from build123d import *

# Parameters (mm, degrees)
F0_R     = 9
F0_R_2   = 4.25
F1_DEPTH = 10
F2_SIZE2 = 0.3639702343
F2_SIZE  = 1
F3_SIZE2 = 0.3639702343
F3_SIZE  = 1
F4_SIZE2 = 0.3639702343
F4_SIZE  = 1
F5_SIZE2 = 0.3639702343
F5_SIZE  = 1


with BuildPart() as f1:
    # F0 (on Top) → F1 (new body)
    with BuildSketch(Plane.XY):
        Circle(F0_R)
        Circle(F0_R_2, mode=Mode.SUBTRACT)
    extrude(amount=F1_DEPTH)

    # F2
    f2_edges = [f1.edges().sort_by_distance(p)[0] for p in [
        (-4.25, 0, 10),
    ]]
    f2_side = f1.faces().sort_by_distance((-4.25, 0, 5))[0]
    chamfer(f2_edges, length=F2_SIZE, length2=F2_SIZE2, reference=f2_side)

    # F3
    f3_edges = [f1.edges().sort_by_distance(p)[0] for p in [
        (-9, 0, 10),
    ]]
    f3_side = f1.faces().sort_by_distance((-9, 0, 5))[0]
    chamfer(f3_edges, length=F3_SIZE, length2=F3_SIZE2, reference=f3_side)

    # F4
    f4_edges = [f1.edges().sort_by_distance(p)[0] for p in [
        (-9, 0, 0),
    ]]
    f4_side = f1.faces().sort_by_distance((-9, 0, 4.5))[0]
    chamfer(f4_edges, length=F4_SIZE, length2=F4_SIZE2, reference=f4_side)

    # F5
    f5_edges = [f1.edges().sort_by_distance(p)[0] for p in [
        (-4.25, 0, 0),
    ]]
    f5_side = f1.faces().sort_by_distance((-8.391766, 0, 0))[0]
    chamfer(f5_edges, length=F5_SIZE, length2=F5_SIZE2, reference=f5_side)


solid = f1.part
Part model, mm, in its own coordinate system. Coordinates: 2 decimals unless noted, no trailing zeros. Order: outer loops, then holes, each group sorted by start corner. A loop starts at its lowest first (then second) coordinate and runs counter-clockwise, first axis right, second up. Notation, with made-up numbers: M -24.5,26.5 L 2.5,26.5 A16 ccw 2.5,30.5 Z; hole C 25.5,53 d1. An arc over 180 degrees is marked long. Use a Markdown table: item, result.
(1) Cut at A-A on y = 0. Write the cut outline in (x, z).
A:
| item | result |
|---|---|
| outline | M -9,1 L -8.64,0 L -5.25,0 L -4.25,0.36 L -4.25,9 L -4.61,10 L -8.64,10 L -9,9 Z; M 4.25,0.36 L 5.25,0 L 8.64,0 L 9,1 L 9,9 L 8.64,10 L 4.61,10 L 4.25,9 Z |
(2) Cut at C-C on z = 1.75. Write the cut outline in (x, y).
A:
| item | result |
|---|---|
| outline | C 0,0 d18; hole C 0,0 d8.5 |
(3) Pull direction X, two halves, no side cores. Call faces 1 (the cylindrical face through (2.285, 3.584, 4.622)), 2 (the cylindrical face through (-1.172, 8.923, 4.944)), 3 (the flat face through (4, -4, 0)): released by +X, released by -X, zero draft, split by the parting line, or undercut.
A:
| item | result |
|---|---|
| face 1 | undercut |
| face 2 | split by the parting line |
| face 3 | zero draft |
(4) Flat gauge pins, fed straight in: pin 1 (6 mm diameter, centred on y = -4, z = 7.5, fed in from -X); pin 2 (1 mm diameter, centred on y = 6.5, z = 6.5, fed in from -X); pin 3 (4 mm diameter, centred on x = 3, z = 3.5, fed in from -Y). Where does each tip first touch, or does it go through?
A:
| item | result |
|---|---|
| pin 1 | stops at x = -8.94 |
| pin 2 | stops at x = -6.71 |
| pin 3 | stops at y = -8.94 |
(5) Probe L1, parallel to Y at x = 0, z = 2.5; L2, parallel to X at y = 1.75, z = 3.75; L3, parallel to X at y = -0.75, z = 4.5. List the from-to ranges inside material, lowest first.
A:
| item | result |
|---|---|
| L1 | y = -9 to -4.25, 4.25 to 9 |
| L2 | x = -8.83 to -3.87, 3.87 to 8.83 |
| L3 | x = -8.97 to -4.18, 4.18 to 8.97 |
